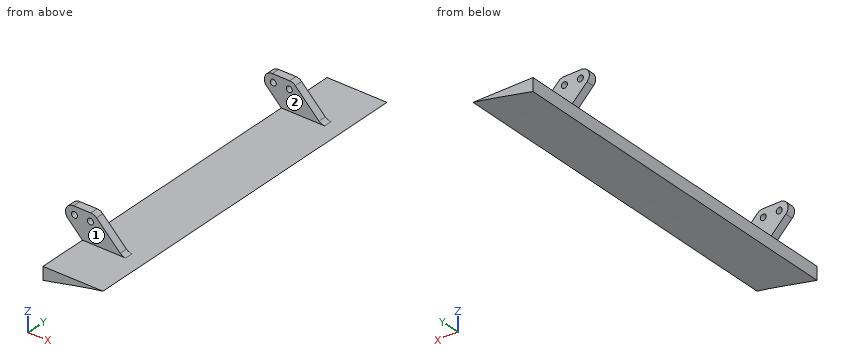
from build123d import *

# Parameters (mm, degrees)
BOSS_EXTRUDE1_DEPTH = 100
CUT_EXTRUDE4_DEPTH  = 100
SKETCH4_W           = 10
SKETCH4_H           = 2
BOSS_EXTRUDE2_DEPTH = 10
FILLET2_R           = 2
SKETCH6_R           = 0.75
CUT_EXTRUDE5_DEPTH  = 110


with BuildPart() as part:
    # Sketch1 → Boss-Extrude1 (new body)
    with BuildSketch(Plane(origin=(0, 0, 0), x_dir=(1, 0, 0), z_dir=(0, 1, 0))):
        with BuildLine():
            Line((-23.835160585, 0), (26.164839415, 0))
            add(Edge.make_bspline(
                [(-24.267578895, 1.256220546), (-22.278212262, 3.553586128), (-18.738393104, 4.793268312), (-8.850120496, 5.774851838), (4.13271293, 5.525012752), (19.211918986, 1.162580188), (26.164839415, 0)],
                knots=[0.021997225, 0.021997225, 0.021997225, 0.021997225, 0.155271246, 0.206186057, 0.531145331, 1, 1, 1, 1], degree=3))
            add(Edge.make_bspline(
                [(-24.267578895, 1.256220546), (-25.367081291, 0.124338635), (-23.835160585, 0)],
                knots=[0, 0, 0, 1, 1, 1], degree=2))
        make_face()
    extrude(amount=BOSS_EXTRUDE1_DEPTH)

    # Sketch2 → Cut-Extrude4 (cut)
    with BuildSketch(Plane.XY.offset(10)):
        Polygon((26.164839415, 95), (11.164839415, 95), (11.164839415, 5), (26.164839415, 5), (26.164839415, 0), (-24.726990199, 0), (-24.726990199, 100), (26.164839415, 100), align=None)
    extrude(amount=-CUT_EXTRUDE4_DEPTH, mode=Mode.SUBTRACT)

    # Sketch4 → Boss-Extrude2 (add, along a direction that is not the sketch's normal)
    with BuildSketch(Plane.XY):
        with Locations((16.164839415, 81.5)):
            Rectangle(SKETCH4_W, SKETCH4_H)
        with Locations((16.164839415, 18.5)):
            Rectangle(SKETCH4_W, SKETCH4_H)
    extrude(amount=BOSS_EXTRUDE2_DEPTH, dir=(-0.7071067811865557, 0, 0.7071067811865395))

    # Fillet2
    fillet2_edges = [part.edges().sort_by_distance(p)[0] for p in [
        (21.164839415, 18.5, 0),
        (14.093771603, 18.5, 7.071067812),
        (4.093771603, 18.5, 7.071067812),
        (21.164839415, 81.5, 0),
        (14.093771603, 81.5, 7.071067812),
        (4.093771603, 81.5, 7.071067812),
    ]]
    fillet(fillet2_edges, radius=FILLET2_R)

    # Sketch6 → Cut-Extrude5 (cut)
    with BuildSketch(Plane(origin=(0, 82.5, 0), x_dir=(1, 0, 0), z_dir=(0, 1, 0))):
        with Locations(Location((9.164839415, -5.071067812, 0), (0, 0, 270))):
            Circle(SKETCH6_R)
        with Locations(Location((13.164839415, -5.071067812, 0), (0, 0, 270))):
            Circle(SKETCH6_R)
    extrude(amount=-CUT_EXTRUDE5_DEPTH, mode=Mode.SUBTRACT)


solid = part.part
Geometry: final body of the model. Coordinates: model frame, mm. Face numbers are marked on the shaded views. Coordinates: 2 decimals unless noted, no trailing zeros. Write each loop counter-clockwise with the first axis right and the second up, starting at its lowest first coordinate (ties: lowest second). Pieces come first, ordered by that corner, then holes. Notation, with made-up numbers: (66, 83) - (115, 83) arc R11 cw to (115, 95) - close; hole circle Ø10 at (-15.75, 13). An arc over 180 degrees is marked (long way). Return JSON: item names as keys, results as strings.
Item 1: Pin query (flat end, axial travel): pin 1 Ø4 at (x, y) = (17, 58.5) entering from -Z; pin 2 Ø2 at (x, z) = (9.16, 5.07) entering from +Y; pin 3 Ø1 at (y, z) = (63.5, -1.5) entering from -X. Return the tip coordinate at first contact, or that it passes through.
Completed:
{"pin 1": "stops at z = -2.37", "pin 2": "stops at y = 82.5", "pin 3": "stops at x = 11.16"}
Item 2: Pull-direction query (Y, two-part tool) for the marked faces 1 and 2; classes: +Y half, -Y half, draft (parallel to the pull), parting line (faces both ways), or undercut.
Completed:
{"face 1": "-Y half", "face 2": "undercut"}
Item 3: Section query A-A (z = 1.5). Output: boundary loops of the cut face in (x, y).
Completed:
{"outline": "(9.66, 17.5) - (19.66, 17.5) - (19.66, 19.5) - (9.66, 19.5) - close; (9.66, 80.5) - (19.66, 80.5) - (19.66, 82.5) - (9.66, 82.5) - close"}
Item 4: Line query: L1, parallel to Y at x = 13.75, z = 6.5; L2, parallel to Z at x = 13.25, y = 62; L3, parallel to Z at x = 15.25, y = 50. Output: solid intervals per line, ascending.
Completed:
{"L1": "y = 17.5 to 19.5, 80.5 to 82.5", "L2": "z = -2.76 to 0", "L3": "z = -2.31 to 0"}
